Can you work these out from the model? Positions are in its coordinate system, mm. A direction names the side the tool comes from. Give positions to 0.01 mm unless a question says otherwise; leave off trailing zeros. Write each loop counter-clockwise with the first axis right and the second up, starting at its lowest first coordinate (ties: lowest second). Pieces come first, ordered by that corner, then holes.
Autodesk Inventor part; units mm, degrees
ref_plane "YZ Plane" through (0, 0, 0) normal (1, 0, 0) x (0, 1, 0)
ref_plane "XZ Plane" through (0, 0, 0) normal (0, 1, 0) x (-1, 0, 0)
ref_plane "XY Plane" through (0, 0, 0) normal (0, 0, 1) x (1, 0, 0)
sketch "Sketch1" plane through (0, 0, 0) normal (0, 1, 0) x (-1, 0, 0)
  line L0 (0, 0) -> (24, 0)
  line L1 (12, 0) -> (12, -5)
  circle A0 centre (12, -5) radius 2.125
  dimension "d0" = 24
  dimension "d1" = 5
  dimension "d2" = 4.25
sketch "Sketch2" plane through (0, 0, 0) normal (0, 1, 0) x (-1, 0, 0)
  line L0 (24, 0) -> (24, 30)
  line L1 (24, 30) -> (0, 30)
  line L2 (0, 0) -> (0, -12.5)
  line L3 (0, -12.5) -> (24, -12.5)
  line L4 (24, -12.5) -> (24, 0)
  line L5 (0, 25) -> (0, 0)
  line L6 (0, 25) -> (-29.86, 25)
  line L7 (0, 30) -> (-29.86, 30)
  line L8 (-29.86, 30) -> (-29.86, 25)
  dimension "d3" = 24
  dimension "d4" = 30
  dimension "d5" = 12.5
  dimension "d6" = 5
  dimension "d20" = 29.86
extrude "Extrusion1" add sketch "Sketch2" along normal blind 8
extrude "Extrusion2" cut sketch "Sketch1" along normal through all
pattern_linear "Rectangular Pattern1" count 2 spacing 6 along (1, 0, 0) count 2 spacing 6 along (-1, 0, 0) of "Extrusion2"
sketch "Sketch4" plane through (-24, 0, -12.5) normal (-1, 0, 0) x (0, 0, 1)
  point P0 (12.5, 0)
sketch "Sketch5" plane through (0, 8, 0) normal (0, 1, 0) x (1, 0, 0)
  line L0 (0, 0) -> (0, 12.5)
  line L1 (0, 12.5) -> (-24, 12.5)
  line L2 (-24, 12.5) -> (-24, 0)
  line L3 (-24, 0) -> (0, 0)
  line L4 (0, -25) -> (0, 12.5)
extrude "Extrusion3" cut sketch "Sketch5" against normal blind 5
sketch "Sketch6" plane through (0, 8, 0) normal (0, 1, 0) x (1, 0, 0)
  line L0 (13.1425, -25) -> (13.1425, 25)
  circle A0 centre (-12, 5) radius 2.125
  line L1 (-12, 5) -> (-12, 23)
  circle A1 centre (-12, 23) radius 10
  line L2 (21.1928, 30) -> (23.1928, 30)
  line L3 (0, 35) -> (20, 35)
  line L4 (20, 35) -> (30.8046, 35) construction
  line L5 (20, 35) -> (37.0437, 35) construction
  line L6 (20, 35) -> (24.8301, 36.2923)
  line L7 (17.3205, 25) -> (22.3205, 25) construction
  line L8 (17.3205, 25) -> (12.3205, 25)
  line L9 (-2, 23) -> (0, 35)
  line L10 (-22, 23) -> (-22, 41)
  line L11 (-22, 41) -> (30, 41)
  line L12 (30, 41) -> (24.8301, 36.2923)
  point P0 (0, 0)
  dimension "d23" = 50
  dimension "d25" = 18
  dimension "d26" = 20
  dimension "d42" = 2
  dimension "d45" = 20
  dimension "d47" = 20
  dimension "d52" = 5
  dimension "d63" = 5
  dimension "d66" = 52
  dimension "d67" = 18
sketch "Sketch7" plane through (0, 0, 0) normal (0, -1, 0) x (1, 0, 0)
  circle A0 centre (-12, -5) radius 2.125
  line L0 (-12, -5) -> (-12, -23)
  circle A1 centre (-12, -23) radius 10
  line L1 (-22, -23) -> (-22, -41)
  line L2 (-22, -41) -> (30, -41)
  line L3 (0, -34.9999) -> (20, -34.9999)
  line L4 (20, -34.9999) -> (24.851, -36.2115)
  line L5 (24.851, -36.2115) -> (30, -41)
  line L6 (0, -34.9999) -> (-2, -23)
  point P0 (0, 0)
  dimension "d27" = 18
  dimension "d28" = 20
  dimension "d68" = 18
  dimension "d69" = 52
  dimension "d70" = 20
  dimension "d71" = 5
extrude "Extrusion4" add sketch "Sketch7" against normal blind 3 contours A1
sketch "Sketch8" plane through (-12, 3, -23) normal (0, 1, 0) x (1, 0, 0)
  circle A0 centre (0, 0) radius 2.125
  point P0 (12, -23)
  dimension "d31" = 4.25
extrude "Extrusion5" cut sketch "Sketch8" against normal blind 1
sketch "Sketch9" plane through (-12, 3, -23) normal (0, 1, 0) x (1, 0, 0)
  line L0 (0, 0) -> (-6, 0)
  circle A0 centre (-6, 0) radius 2.125
  point P0 (12, -23)
  dimension "d34" = 6
  dimension "d35" = 4.25
extrude "Extrusion6" cut sketch "Sketch9" against normal through all
pattern_circular "Circular Pattern1" count 4 over 360 about axis through (-12, 0, -23) along (0, 1, 0) of "Extrusion6"
sketch "Sketch10" plane through (-12, 0, -23) normal (0, -1, 0) x (1, 0, 0)
  circle A0 centre (0, 0) radius 10
  line L0 (-10, 0) -> (-10, -18)
  line L1 (-10, -18) -> (42, -18)
  line L2 (12, -12) -> (32, -12)
  line L3 (32, -12) -> (36.8295, -13.2918)
  line L4 (36.8295, -13.2918) -> (42, -18)
  arc A1 (-10, 0) -> (10, 0) centre (0, 0) ccw
  line L5 (10, 0) -> (12, -12)
  point P0 (12, 23)
  dimension "d72" = 18
  dimension "d73" = 52
  dimension "d74" = 20
extrude "Extrusion7" add sketch "Sketch10" against normal blind 8 contours L5 L2 L3 L4 L1 L0 A0
sketch "Sketch11" plane through (0, 0, 25) normal (1, 0, 0) x (0, 0, -1)
  line L0 (25, 8) -> (37.5, 8)
  line L1 (37.5, 8) -> (37.5, 4)
  line L2 (37.5, 4) -> (25, 4)
  line L3 (25, 4) -> (25, 8)
  point P0 (25, 0)
  dimension "d77" = 4
extrude "Extrusion8" add sketch "Sketch11" against normal blind 24
sketch "Sketch12" plane through (0, 8, 0) normal (0, 1, 0) x (1, 0, 0)
  circle A0 centre (-12, 5) radius 2.125
  circle A1 centre (-12, 5) radius 2.125
  point P0 (0, 0)
  dimension "d80" = 4.25
extrude "Extrusion9" cut sketch "Sketch12" against normal through all
pattern_linear "Rectangular Pattern2" count 3 spacing 6 along (1, 0, 0) of "Extrusion9"
sketch "Sketch13" plane through (0, 8, 0) normal (0, 1, 0) x (1, 0, 0)
  line L0 (30, 41) -> (29.8598, -25)
  point P0 (0, 0)
  point P1 (29.86, -25)
fillet "Fillet1" radius 5 1 edges at (29.86, 4, 30)
sketch "Sketch14" plane through (0, 0, 25) normal (1, 0, 0) x (0, 0, -1)
  line L0 (37.5, 3) -> (25, 3)
  line L1 (25, 3) -> (25, 0)
  line L2 (25, 0) -> (37.5, 0)
  line L3 (37.5, 0) -> (37.5, 3)
  line L4 (37.5, 0) -> (66, 0)
  line L5 (66, 0) -> (66, 8)
  line L6 (66, 8) -> (37.5, 8)
  line L7 (37.5, 8) -> (37.5, 0)
sketch "Sketch15" plane through (0, 0, 25) normal (1, 0, 0) x (0, 0, -1)
  point P0 (25, 0)
sketch "Sketch16" plane through (-24, 0, -12.5) normal (-1, 0, 0) x (0, 0, 1)
  line L0 (0, 8) -> (42.5, 8)
  line L1 (0, 4) -> (12.5, 4)
  line L2 (12.5, 4) -> (12.5, 8)
  line L3 (12.5, 8) -> (0, 8)
  line L4 (0, 8) -> (0, 4)
  line L5 (-0.5, 0) -> (-10.5, 0)
  line L6 (-0.5431, 0) -> (-28.5, 0)
  line L7 (-28.5, 0) -> (-28.5, 8)
  line L8 (-28.5, 8) -> (-0.5431, 8)
  line L9 (-0.5431, 8) -> (-0.5431, 0)
  point P0 (12.5, 0)
sketch "Sketch17" plane through (0, 8, 0) normal (0, 1, 0) x (1, 0, 0)
  line L0 (-28.6904, -36.0385) -> (31.2177, -36.0385)
  line L1 (31.2177, -36.0385) -> (31.2177, 12.5)
  line L2 (31.2177, 12.5) -> (-28.6904, 12.5)
  line L3 (-28.6904, 12.5) -> (-28.6904, -36.0385)
  point P0 (0, 0)
extrude "Extrusion10" cut sketch "Sketch17" against normal through all
sketch "Sketch18" plane through (-12, 8, -23) normal (0, 1, 0) x (1, 0, 0)
  line L0 (12, 12) -> (12, 14)
  line L1 (12, 14) -> (-10, 14)
  line L2 (-10, 14) -> (-10, 0)
  line L3 (-10, 0) -> (12, 0)
  line L4 (12, 0) -> (12, 14)
  point P0 (12, -23)
  dimension "d89" = 2
extrude "Extrusion11" cut sketch "Sketch18" against normal blind 5
sketch "Sketch19" plane through (-22, 0, -41) normal (-1, 0, 0) x (0, 0, 1)
  line L0 (0, 0) -> (-2, 0)
  line L1 (-2, 0) -> (-2, 8)
  line L2 (-2, 8) -> (0, 8)
  line L3 (0, 8) -> (0, 0)
  point P0 (41, 0)
  dimension "d92" = 2
extrude "Extrusion12" add sketch "Sketch19" against normal blind 20
sketch "Sketch20" plane through (-12, 8, -23) normal (0, 1, 0) x (1, 0, 0)
  line L0 (10, 20) -> (42.0506, 20)
  line L1 (42.0506, 20) -> (42.0506, 0.0873)
  line L2 (42.0506, 0.0873) -> (10, 0.0873)
  line L3 (10, 0.0873) -> (10, 20)
  point P0 (12, -23)
extrude "Extrusion13" cut sketch "Sketch20" against normal through all
sketch "Sketch21" plane through (-22, 0, -23) normal (-1, 0, 0) x (0, 0, 1)
  line L0 (-20, 0) -> (-14, 0)
  line L1 (-14, 0) -> (-14, 8)
  line L2 (-14, 8) -> (-20, 8)
  line L3 (-20, 8) -> (-20, 0)
  point P0 (23, 0)
extrude "Extrusion14" add sketch "Sketch21" along normal blind 35
sketch "Sketch22" plane through (0, 0, 0) normal (0, -1, 0) x (1, 0, 0)
  point P0 (0, 0)
fillet "Fillet2" radius 6 1 edges at (-57, 4, -37)
sketch "Sketch24" plane through (-12, 8, -23) normal (0, 1, 0) x (1, 0, 0)
  arc A0 (-45, 20) -> (-39, 14) centre (-39, 20) ccw
  line L0 (-39, 14) -> (-36, 14)
  line L1 (-10, 14) -> (-39, 14)
  line L2 (-36, 14) -> (-36, 20)
  line L3 (-45, 20) -> (10, 20)
  point P0 (12, -23)
  dimension "d101" = 3
extrude "Extrusion15" add sketch "Sketch24" along normal blind 15
equation "\"d81\" = d80"
properties part number "CraneGripper"
(1) Imagine slicing it at B-B, the plane x = -18. Write out the boundary of the cut face in (y, z) (3 decimals), plus the area to 3 significant figures.
Returned:
outline: (0, -43) - (8, -43) - (8, -37) - (3, -37) - (3, -25.125) - (0, -25.125) - close; (0, -20.875) - (3, -20.875) - (3, -15) - (0, -15) - close
area: 101 mm2
(2) For faces 5 (the face through (-22, 2, -30)), 6 (the face through (-12.461, 2.507, -20.926)), 7 (the face through (-48, 15, -40)), 8 (the face through (-19.69, 1.52, -21.71)), 9 (the face through (-14, 3, -25)), which set-ups out of +Z, -Z, +X, -X, +Y, -Y let a thin tool reach every point of the face, with its end or its side?
Returned:
face 5: +Z, -X, +Y, -Y
face 6: +Y
face 7: +Z, -Z, +X, +Y
face 8: +Y, -Y
face 9: +Z, +X, -X, +Y
(3) Imagine slicing it at D-D, the plane x = -12. Write out the boundary of the cut face in (y, z) (3 decimals).
Returned:
outline: (0, -43) - (8, -43) - (8, -37) - (3, -37) - (3, -31.125) - (0, -31.125) - close; (0, -26.875) - (3, -26.875) - (3, -25.125) - (2, -25.125) - (2, -20.875) - (3, -20.875) - (3, -19.125) - (0, -19.125) - close; (0, -14.875) - (3, -14.875) - (3, -13) - (0, -13) - close
(4) Will these pins go through, and if not, where does the flat tip stop? P1, Ø10, axis at x = -8.5, y = 17.5, coming from the -Z side; P2, Ø6.5, axis at y = 3, z = -34.5, coming from the +X side; P3, Ø16, axis at x = -12, z = -19, coming from the +Y side; P4, Ø10, axis at y = 7, z = -25, coming from the -X side.
Returned:
P1: passes through
P2: stops at x = -2
P3: stops at y = 3
P4: stops at x = -22
(5) If I drill on L1, parallel to X at y = 1.9, z = -29 (3 decimals); L2, parallel to Y at x = -15, z = -36.25; L3, parallel to Y at x = -12.5, z = -21.5, over which ranges is the centre line in solid material (lowest first)?
Returned:
L1: x = -22 to -14.125, -9.875 to -2
L2: y = 0 to 3
L3: y = 0 to 2
(6) If we mould it in two halves opening along Z, with no side actions, what happens to faces 1 (the face through (-52, 23, -40)), 2 (the face through (-55.196, 15.395, -38.711)), 3 (the face through (-12.814, 1.521, -27.037)), 4 (the face through (-12.093, 1.521, -14.877))? For each: +Z half, -Z half, draft (parallel to the pull), parting line (faces both ways), or undercut.
Returned:
face 1: draft
face 2: +Z half
face 3: undercut
face 4: undercut
(7) Imagine slicing it at C-C, the plane z = -21.5. Write out the boundary of the cut face in (x, y), plus the area to 3 significant figures.
Returned:
outline: (-21.89, 0) - (-19.51, 0) - (-19.51, 3) - (-21.89, 3) - close; (-16.49, 0) - (-7.51, 0) - (-7.51, 3) - (-10.49, 3) - (-10.49, 2) - (-13.51, 2) - (-13.51, 3) - (-16.49, 3) - close; (-4.49, 0) - (-2.11, 0) - (-2.11, 3) - (-4.49, 3) - close
area: 38.2 mm2
(8) Imagine slicing it at A-A, the plane z = -29. Write out the boundary of the cut face in (x, y) (3 decimals), plus the area to 4 significant figures.
Returned:
outline: (-22, 0) - (-14.125, 0) - (-14.125, 3) - (-22, 3) - close; (-9.875, 0) - (-2, 0) - (-2, 3) - (-9.875, 3) - close
area: 47.25 mm2
